Can you work these out from the model? Positions are in its coordinate system, mm. Give positions to 0.01 mm unless a question says otherwise; leave off trailing zeros. Write each loop counter-clockwise with the first axis right and the second up, starting at its lowest first coordinate (ties: lowest second). Pieces come first, ordered by that corner, then holes.
1. I'm going to push flat-ended pins straight in: pin 1 (12 mm diameter, centred on x = 2.5, z = 1, fed in from -Y); pin 2 (2 mm diameter, centred on x = -2, z = 3.5, fed in from +Y); pin 3 (1 mm diameter, centred on x = -2, y = -0.5, fed in from -Z). Where does each tip first touch, or does it pass through?
2. Suppose I cut it at A-A (y = 0.25). Please give me the cut outline in (x, z).
3. Suppose I cut it at D-D (x = -2.54). Please give me the cut outline in (y, z).
4. Suppose I cut it at C-C (z = 0). Please give me the cut outline in (x, y).
5. Suppose I cut it at B-B (x = 5.08). Please give me the cut outline in (y, z).
6. If I drill on probe 1 along X at (y, z) = (-0.1, 9.5); probe 2 along Y at (x, z) = (-3, 4.25); probe 3 along X at (y, z) = (0.2, -7.75), over which ranges is the centre line in solid material (lowest first)?
```python
from build123d import *

# Parameters (mm, degrees)
SCHIZZO1_R                   = 12
ESTRUSIONE_ESTRUSIONE1_DEPTH = 0.8
SCHIZZO2_R                   = 0.45
TAGLIO_ESTRUSIONE1_DEPTH     = 18.045820602
SCHIZZO3_R                   = 0.75
SCHIZZO3_R_2                 = 0.45
ESTRUSIONE_ESTRUSIONE2_DEPTH = 0.05


with BuildPart() as part:
    # Schizzo1 → Estrusione-Estrusione1 (new, symmetric)
    with BuildSketch(Plane(origin=(0, 0, 0), x_dir=(1, 0, 0), z_dir=(0, 1, 0))):
        with Locations(Location((0, 0, 0), (0, 0, 270))):
            Circle(SCHIZZO1_R)
    extrude(amount=ESTRUSIONE_ESTRUSIONE1_DEPTH, both=True)

    # Schizzo2 → Taglio-Estrusione1 (cut, through all)
    with BuildSketch(Plane(origin=(0, 0.8, 0), x_dir=(1, 0, 0), z_dir=(0, 1, 0))):
        with Locations(Location((0, -9.5, 0), (0, 0, 270))):
            Circle(SCHIZZO2_R)
        with Locations(Location((2.54, -9.5, 0), (0, 0, 270))):
            Circle(SCHIZZO2_R)
        with Locations(Location((5.08, -9.5, 0), (0, 0, 270))):
            Circle(SCHIZZO2_R)
        with Locations(Location((-2.54, -9.5, 0), (0, 0, 270))):
            Circle(SCHIZZO2_R)
        with Locations(Location((-5.08, -9.5, 0), (0, 0, 270))):
            Circle(SCHIZZO2_R)
    extrude(amount=-TAGLIO_ESTRUSIONE1_DEPTH, mode=Mode.SUBTRACT)

    # Schizzo3 → Estrusione-Estrusione2 (add, symmetric)
    # profile 1 of 5: a face of its own
    with BuildSketch(Plane(origin=(0, 0.8, 0), x_dir=(1, 0, 0), z_dir=(0, 1, 0))):
        with Locations(Location((-5.08, -9.5, 0), (0, 0, 270))):
            Circle(SCHIZZO3_R)
        with Locations(Location((-5.08, -9.5, 0), (0, 0, 270))):
            Circle(SCHIZZO3_R_2, mode=Mode.SUBTRACT)
    # profile 2 of 5: a face of its own
    with BuildSketch(Plane(origin=(0, 0.8, 0), x_dir=(1, 0, 0), z_dir=(0, 1, 0))):
        with Locations(Location((-2.54, -9.5, 0), (0, 0, 270))):
            Circle(SCHIZZO3_R)
        with Locations(Location((-2.54, -9.5, 0), (0, 0, 270))):
            Circle(SCHIZZO3_R_2, mode=Mode.SUBTRACT)
    # profile 3 of 5: a face of its own
    with BuildSketch(Plane(origin=(0, 0.8, 0), x_dir=(1, 0, 0), z_dir=(0, 1, 0))):
        with Locations(Location((0, -9.5, 0), (0, 0, 270))):
            Circle(SCHIZZO3_R)
        with Locations(Location((0, -9.5, 0), (0, 0, 270))):
            Circle(SCHIZZO3_R_2, mode=Mode.SUBTRACT)
    # profile 4 of 5: a face of its own
    with BuildSketch(Plane(origin=(0, 0.8, 0), x_dir=(1, 0, 0), z_dir=(0, 1, 0))):
        with Locations(Location((2.54, -9.5, 0), (0, 0, 270))):
            Circle(SCHIZZO3_R)
        with Locations(Location((2.54, -9.5, 0), (0, 0, 270))):
            Circle(SCHIZZO3_R_2, mode=Mode.SUBTRACT)
    # profile 5 of 5: a face of its own
    with BuildSketch(Plane(origin=(0, 0.8, 0), x_dir=(1, 0, 0), z_dir=(0, 1, 0))):
        with Locations(Location((5.08, -9.5, 0), (0, 0, 270))):
            Circle(SCHIZZO3_R)
        with Locations(Location((5.08, -9.5, 0), (0, 0, 270))):
            Circle(SCHIZZO3_R_2, mode=Mode.SUBTRACT)
    estrusione_estrusione2 = extrude(amount=ESTRUSIONE_ESTRUSIONE2_DEPTH, both=True)

    # Specchia1: Estrusione-Estrusione2 across plane
    add(estrusione_estrusione2.mirror(Plane.ZX))


solid = part.part
```
Checks:
1. pin 1: stops at y = -0.8
1. pin 2: stops at y = 0.8
1. pin 3: stops at z = -11.91
2. outline: circle Ø24 at (0, 0); hole circle Ø0.9 at (-5.08, 9.5); hole circle Ø0.9 at (-2.54, 9.5); hole circle Ø0.9 at (0, 9.5); hole circle Ø0.9 at (2.54, 9.5); hole circle Ø0.9 at (5.08, 9.5)
3. outline: (-0.85, 8.75) - (-0.8, 8.75) - (-0.8, -11.73) - (0.8, -11.73) - (0.8, 8.75) - (0.85, 8.75) - (0.85, 9.05) - (-0.85, 9.05) - close; (-0.85, 9.95) - (0.85, 9.95) - (0.85, 10.25) - (0.8, 10.25) - (0.8, 11.73) - (-0.8, 11.73) - (-0.8, 10.25) - (-0.85, 10.25) - close
4. outline: (-12, -0.8) - (12, -0.8) - (12, 0.8) - (-12, 0.8) - close
5. outline: (-0.85, 8.75) - (-0.8, 8.75) - (-0.8, -10.87) - (0.8, -10.87) - (0.8, 8.75) - (0.85, 8.75) - (0.85, 9.05) - (-0.85, 9.05) - close; (-0.85, 9.95) - (0.85, 9.95) - (0.85, 10.25) - (0.8, 10.25) - (0.8, 10.87) - (-0.8, 10.87) - (-0.8, 10.25) - (-0.85, 10.25) - close
6. probe 1: x = -7.33 to -5.53, -4.63 to -2.99, -2.09 to -0.45, 0.45 to 2.09, 2.99 to 4.63, 5.53 to 7.33
6. probe 2: y = -0.8 to 0.8
6. probe 3: x = -9.16 to 9.16
